The figure shows three views and two pictorial views of one solid part (mm, origin at its lowest corner). Answer the questions. A direction names the side the tool comes from. Give positions to 0.01 mm unless a question says otherwise; leave off trailing zeros. Loops run counter-clockwise (first coordinate to the right, second up) from the corner with the lowest first, then second, coordinate; pieces in that order, holes last. Notation, with made-up numbers: M 72,-14 L 116,-14 A7 ccw 116,-5 Z; hole C 41,56.25 d6. An arc over 180 degrees is marked long. Answer in a Markdown table with one row per item. Add a question column.
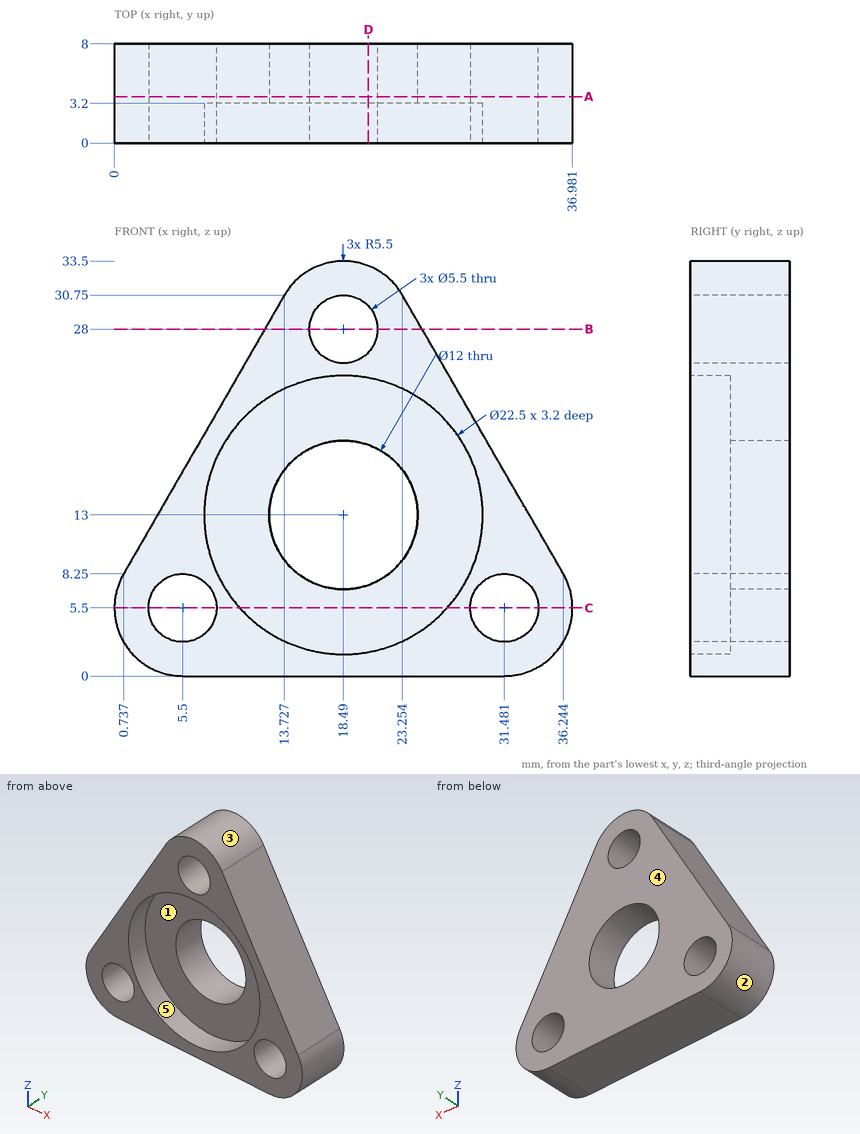
(1) The mould has two halves that part along X. Classify the marked faces 3, 4 and 5: pulls with the +X half, pulls with the -X half, needs draft (parallel to the pull), parting line crosses it, or undercut.
(2) Consider line 1 along X through (y, z) = (5, 5) (1 decimal); line 2 along X through (y, z) = (5.75, 4) (1 decimal); line 3 along Y through (x, z) = (21, 19). Determine where each line is inside the solid, lowest interval first. Write a range as from..to.
(3) Section B-B, the plane z = 28 is taken. Determine the outline of the cut face in (x, y).
(4) Which of the six approach directions +Z, -Z, +X, -X, +Y, -Y give full straight-line access (tool end or side, diameter ignored) to the marked faces 1 and 2?
(5) Each of these flat-tipped pins is pushed along its axis until it touches: P1, Ø2, axis at y = 5.5, z = 24.5, coming from the +X side; P2, Ø1, axis at x = 33, y = 2.5, coming from the -Z side (1 decimal); P3, Ø1, axis at x = 19.5, y = 7, coming from the +Z side. Where does it stop, or does it pass through?
(6) Section C-C, the plane z = 5.5 is taken. State how many separate pieces and enclosed holes the cut face has, and give its area (3 significant figures).
(7) Section D-D, the plane x = 20.5 is taken. Determine the outline of the cut face in (y, z), and give its area (3 significant figures).
(8) Section A-A, the plane y = 3.75 is taken. Determine the outline of the cut face in (x, z).
Numbers:
| question | item | result |
|---|---|---|
| 1 | face 3 | parting line crosses it |
| 1 | face 4 | needs draft |
| 1 | face 5 | undercut |
| 2 | line 1 | x = 0..2.8, 8.2..28.8, 34.2..37 |
| 2 | line 2 | x = 0.2..3.2, 7.8..29.2, 33.8..36.8 |
| 2 | line 3 | y = 3.2..8 |
| 3 | outline | M 12.14,0 L 15.74,0 L 15.74,8 L 12.14,8 Z; M 21.24,0 L 24.84,0 L 24.84,8 L 21.24,8 Z |
| 4 | face 1 | -Y |
| 4 | face 2 | -X, +Y, -Y |
| 5 | P1 | stops at x = 27.44 |
| 5 | P2 | stops at z = 0.1 |
| 5 | P3 | stops at z = 33.48 |
| 6 | separate pieces | 3 |
| 6 | enclosed holes | 0 |
| 6 | area | 154 mm² |
| 7 | outline | M 0,0 L 8,0 L 8,7.35 L 3.2,7.35 L 3.2,1.93 L 0,1.93 Z; M 0,24.07 L 3.2,24.07 L 3.2,18.65 L 8,18.65 L 8,26.12 L 0,26.12 Z; M 0,29.88 L 8,29.88 L 8,33.12 L 0,33.12 Z |
| 7 | area | 110 mm² |
| 8 | outline | M 0.74,8.25 A5.5 ccw 5.5,0 L 31.48,0 A5.5 ccw 36.24,8.25 L 23.25,30.75 A5.5 ccw 13.73,30.75 Z; hole C 5.5,5.5 d5.5; hole C 18.49,13 d12; hole C 18.49,28 d5.5; hole C 31.48,5.5 d5.5 |
